```python
from build123d import *


with BuildPart() as f2:
    # F2: sweep along a path in F0
    with BuildLine(Plane.XY) as f2_path:
        Line((-143.7282372266, -156.79862791), (156.2717627734, -156.79862791))
        Line((156.2717627734, -156.79862791), (156.2717627734, 143.20137209))
        Line((156.2717627734, 143.20137209), (-143.7282372266, 143.20137209))
        Line((-143.7282372266, 143.20137209), (-143.7282372266, -156.79862791))
    # F1 (on Right) → F2 (sweep)
    with BuildSketch(Plane.YZ):
        Polygon((-152.8481326103, -0.3476490092), (-144.8981165886, -0.3476490092), (-144.8981165886, 2.6523509908), (-147.8981165886, 2.6523509908), (-147.8981165886, 5.6523509908), (-144.6481214636, 5.6523509908), (-144.6481214636, 15.0182117835), (-156.8481326103, 15.0182117835), (-156.8481326103, 3.6523509908), (-152.8481326103, 3.6523509908), align=None)
    sweep(path=f2_path.line, transition=Transition.RIGHT)


solid = f2.part
```
Model file for the job. Use its own axes, mm. A direction names the side the tool comes from. Give positions to 0.01 mm unless a question says otherwise; leave off trailing zeros. Write each loop counter-clockwise with the first axis right and the second up, starting at its lowest first coordinate (ties: lowest second). Pieces come first, ordered by that corner, then holes. Notation, with made-up numbers: (-14, -14) - (16, -14) arc R30 ccw to (16, 12) - close; hole circle Ø6 at (76, -12.5). An arc over 180 degrees is marked (long way). One line per question, with ' | ' between items. Start each with the question number.
(1) Wall check: line 1 along X through (y, z) = (-39.5, 1.75); line 2 along Y through (x, z) = (-64, 11); line 3 along X through (y, z) = (-111.5, 5.25). Give the ranges that are in metal, low to high. Write a range as from..to.
(2) Slice it at A-A on y = 66. Write the cut outline in (x, z).
(3) 3-axis set-ups, long thin cutter, end or side, ignore diameter. For faces 5 (the face through (4, 131.051, 10)), 6 (the face through (156.321, -5, 9)): which of +Z, -Z, +X, -X, +Y, -Y reach the whole face in a straight line?
(4) Two-plate mould, pull along Y, no slides. Class faces 1 (the face through (4, 143.251, 9)), 2 (the face through (8, -156.848, 9)), 3 (the face through (-131.578, -9, 10)), 4 (the face through (-138, 5, 15.018)): +Y half, -Y half, draft (parallel to the pull), parting line (faces both ways), or undercut.
(5) Pin check, flat tips, straight feed: P1, Ø1.2, axis at x = 61, z = 1.5, coming from the +Y side; P2, Ø2, axis at y = 16, z = 2, coming from the +X side; P3, Ø4.5, axis at x = 0, z = 1, coming from the -Y side. Stop position of each tip, or through.
(6) Slice it at B-B on z = 8.75. Write the cut outline in (x, y).
(7) Slice it at C-C on x = -7. Write the cut outline in (y, z).
Results below:
1) line 1: -139.78..-131.83, 144.37..152.32 | line 2: -156.85..-144.65, 131.05..143.25 | line 3: -143.78..-134.83, 147.37..156.32
2) outline: (-143.78, 3.65) - (-139.78, 3.65) - (-139.78, -0.35) - (-131.83, -0.35) - (-131.83, 2.65) - (-134.83, 2.65) - (-134.83, 5.65) - (-131.58, 5.65) - (-131.58, 15.02) - (-143.78, 15.02) - close; (144.12, 5.65) - (147.37, 5.65) - (147.37, 2.65) - (144.37, 2.65) - (144.37, -0.35) - (152.32, -0.35) - (152.32, 3.65) - (156.32, 3.65) - (156.32, 15.02) - (144.12, 15.02) - close
3) face 5: +Z, -Z | face 6: +Z, -Z, +X, +Y, -Y
4) face 1: +Y half | face 2: -Y half | face 3: undercut | face 4: draft
5) P1: y = 139.25 | P2: x = 152.32 | P3: y = -152.85
6) outline: (-143.78, -156.85) - (156.32, -156.85) - (156.32, 143.25) - (-143.78, 143.25) - close; hole (-131.58, -144.65) - (144.12, -144.65) - (144.12, 131.05) - (-131.58, 131.05) - close
7) outline: (-156.85, 3.65) - (-152.85, 3.65) - (-152.85, -0.35) - (-144.9, -0.35) - (-144.9, 2.65) - (-147.9, 2.65) - (-147.9, 5.65) - (-144.65, 5.65) - (-144.65, 15.02) - (-156.85, 15.02) - close; (131.05, 5.65) - (134.3, 5.65) - (134.3, 2.65) - (131.3, 2.65) - (131.3, -0.35) - (139.25, -0.35) - (139.25, 3.65) - (143.25, 3.65) - (143.25, 15.02) - (131.05, 15.02) - close
